Work out the finished part from the listing and answer in its coordinate system (mm). A direction names the side the tool comes from. Give positions to 0.01 mm unless a question says otherwise; leave off trailing zeros. Loops run counter-clockwise (first coordinate to the right, second up) from the corner with the lowest first, then second, coordinate; pieces in that order, holes last. Notation, with made-up numbers: (4.25, 34) - (34.25, 34) arc R24 cw to (34.25, 69) - close; hole circle Ø7 at (42.5, 29.5). An arc over 180 degrees is marked (long way). One line per question, with ' | ' between items.
Autodesk Inventor part; units mm, degrees
ref_plane "YZ Plane" through (0, 0, 0) normal (1, 0, 0) x (0, 1, 0)
ref_plane "XZ Plane" through (0, 0, 0) normal (0, 1, 0) x (-1, 0, 0)
ref_plane "XY Plane" through (0, 0, 0) normal (0, 0, 1) x (1, 0, 0)
sketch "Sketch1" plane through (0, 0, 0) normal (0, 1, 0) x (-1, 0, 0)
  circle A0 centre (0, 0) radius 3
  circle A1 centre (0, 0) radius 4.5
  line L0 (0, 0) -> (7.62, 0) construction
  circle A2 centre (0, 0) radius 1.5
  line L1 (0, 0) -> (0, 4.5) construction
  arc A3 (20.25, -2.4875) -> (20.25, 2.4875) centre (20, 0) ccw
  line L2 (20, 0) -> (0, 0)
  arc A4 (-20.25, 2.4875) -> (-20.25, -2.4875) centre (-20, 0) ccw
  line L3 (20.25, 2.4875) -> (0.45, 4.4774)
  line L4 (20.25, -2.4875) -> (0.45, -4.4774)
  line L5 (-20.25, -2.4875) -> (-0.45, -4.4774)
  line L6 (-20.25, 2.4875) -> (-0.45, 4.4774)
  point P0 (10.62, 0)
  point P1 (13.62, 0)
  point P2 (16.62, 0)
  point P3 (19.62, 0)
  point P4 (-7.62, 0)
  point P5 (-7.62, 0)
  point P6 (-10.62, 0)
  point P7 (-13.62, 0)
  point P8 (-16.62, 0)
  point P9 (-19.62, 0)
  dimension "d0" = 6
  dimension "d1" = 9
  dimension "d2" = 7.62
  dimension "d6" = 3
  dimension "d9" = 3
  dimension "d14" = 2.5
  dimension "d15" = 40
extrude "Extrusion1" add sketch "Sketch1" along normal blind 2 contours A1 | A1 L3 A3 L4 | A1 L5 A4 L6
extrude "Extrusion2" add sketch "Sketch1" against normal blind 1 contours A0 | A1
extrude "Extrusion3" add sketch "Sketch1" against normal blind 4 contours A1
hole "Hole1" at (-7.62, 0, 0) at (-10.62, 0, 0) at (-13.62, 0, 0) at (-16.62, 0, 0) at (-19.62, 0, 0) at (19.62, 0, 0) at (16.62, 0, 0) at (13.62, 0, 0) at (10.62, 0, 0) at (7.62, 0, 0) direction (0, 1, 0) diameter 1.2 depth 8 tip angle 118
properties part number "servo arm HK15138 2 cut to 1"
1. Determine the mould class of faces 1 (the cylindrical face through (20.206, 1.014, 0.13)), 2 (the flat face through (12, 0, 0)), 3 (the cylindrical face through (22.5, 1, -0.1)) for opening direction Z: +Z half, -Z half, draft (parallel to the pull), parting line (faces both ways), or undercut.
Evaluation:
face 1: undercut | face 2: draft | face 3: parting line
2. Find section A-A on y = 0.65. State how many separate pieces and enclosed holes the cut face has, then the cut area to 3 significant figures.
Evaluation:
separate pieces: 1 | enclosed holes: 11 | area: 261 mm2
3. Find section D-D on y = -2.35. Write down the section's boundary in (x, z).
Evaluation:
outline: circle Ø9 at (0, 0); hole circle Ø6 at (0, 0)
4. Find section C-C on z = 1. Write down the section's boundary in (x, y).
Evaluation:
outline: (-22.29, 0) - (-4.39, 0) - (-4.39, -4) - (-2.83, -4) - (-2.83, -1) - (-1.12, -1) - (-1.12, 0) - (-2.83, 0) - (-2.83, 2) - (-22.29, 2) - close; (1.12, -1) - (2.83, -1) - (2.83, -4) - (4.39, -4) - (4.39, 0) - (22.29, 0) - (22.29, 2) - (2.83, 2) - (2.83, 0) - (1.12, 0) - close
5. Consider L1, parallel to Y at x = 13, z = 2; L2, parallel to X at y = -1.8, z = 2; L3, parallel to Z at x = -10.62, y = 0.6. Determine where each line is inside the solid, lowest interval first.
Evaluation:
L1: 0 to 2 | L2: -4.03 to -2.24, 2.24 to 4.03 | L3: -3.46 to -0.6, 0.6 to 3.46
6. Find section B-B on x = 0. Write down the section's boundary in (y, z), then the cut area to 3 significant figures.
Evaluation:
outline: (-4, -4.5) - (2, -4.5) - (2, -3) - (0, -3) - (0, -1.5) - (-1, -1.5) - (-1, -3) - (-4, -3) - close; (-4, 3) - (-1, 3) - (-1, 1.5) - (0, 1.5) - (0, 3) - (2, 3) - (2, 4.5) - (-4, 4.5) - close | area: 21.0 mm2
7. Which of the six approach directions +Z, -Z, +X, -X, +Y, -Y give full straight-line access (tool end or side, diameter ignored) to faces 4 (the cylindrical face through (7.025, 1.014, 0.078)), 5 (the flat face through (-1.3, -1, -1.3)), 6 (the cylindrical face through (3, 1, 0))?
Evaluation:
face 4: +Y, -Y | face 5: -Y | face 6: +Y
8. Flat-ended cylindrical pins translate along their axes: pin 1 (1.5 mm diameter, centred on x = -2, y = -2.5, fed in from -Z); pin 2 (2 mm diameter, centred on x = 16, z = -2, fed in from -Y); pin 3 (2 mm diameter, centred on x = -4.5, y = 1, fed in from +Z). Find the tip coordinate at first contact, or state that the pin passes through.
Evaluation:
pin 1: z = -4.32 | pin 2: y = 0 | pin 3: z = 4.17
